Autodesk Inventor part; units mm, degrees
ref_plane "YZ Plane" through (0, 0, 0) normal (1, 0, 0) x (0, 1, 0)
ref_plane "XZ Plane" through (0, 0, 0) normal (0, 1, 0) x (-1, 0, 0)
ref_plane "XY Plane" through (0, 0, 0) normal (0, 0, 1) x (1, 0, 0)
sketch "Sketch1" plane through (0, 0, 0) normal (0, 0, 1) x (1, 0, 0)
  line L0 (0, 0) -> (0, 41.5)
  circle A0 centre (0, 41.5) radius 11
  line L1 (0, 41.5) -> (0, 52.5)
  line L2 (0, 52.5) -> (16, 52.5)
  line L3 (16, 52.5) -> (16, 0)
  line L4 (16, 0) -> (0, 0)
  line L5 (0, 0) -> (-16, 0)
  line L6 (-16, 0) -> (-16, 52.5)
  line L7 (-16, 52.5) -> (0, 52.5)
  dimension "d1" = 22
  dimension "d0" = 41.5
  dimension "d2" = 16
  dimension "d3" = 16
extrude "Extrusion1" add sketch "Sketch1" along normal mid plane 38
extrude "Extrusion2" add sketch "Sketch1" along normal mid plane 42 contours A0 L1 L0 | L0 L1 A0
fillet "Fillet1" radius 2 6 edges at (-16, 26.25, 19) (-16, 26.25, -19) (-16, 52.5, 0) (16, 52.5, 0) (16, 26.25, 19) (16, 26.25, -19)
sketch "Sketch2" plane through (-14, 0, 19) normal (0, -1, 0) x (1, 0, 0)
  circle A0 centre (14, -19) radius 11
  dimension "d9" = 22
extrude "Extrusion3" cut sketch "Sketch2" against normal blind 1
properties part number "Shoulder"
Verification items for the finished model (mm, model axes). A direction names the side the tool comes from. Coordinates: 2 decimals unless noted, no trailing zeros. Write each loop counter-clockwise with the first axis right and the second up, starting at its lowest first coordinate (ties: lowest second). Pieces come first, ordered by that corner, then holes. Notation, with made-up numbers: (24.25, 3) - (81.25, 3) arc R32 ccw to (81.25, 37) - close; hole circle Ø2 at (3, -27.75). An arc over 180 degrees is marked (long way). One line per question, with ' | ' between items. Start each with the question number.
1. Draft check along Z on faces 1 (the cylindrical face through (-15.43, 26.62, 18.4)), 2 (the flat face through (0, 1, 0)), 3 (the cylindrical face through (-15.4, 26.62, -18.43)), 4 (the flat face through (-7, 0, -9)). Enter one of: released by +Z, released by -Z, zero draft, split by the parting line, or undercut.
2. Section check C-C (y = 9.5). Enter the section's corners in (x, z), plus the area to 3 significant figures.
3. Section check A-A (y = 41.5). Enter the section's corners in (x, z).
4. Material ranges on line 1 along Z through (x, y) = (8, 24); line 2 along Y through (x, z) = (8.5, 3); line 3 along X through (y, z) = (41.5, -17.5), recorded low to high.
5. Gauge pin test, flat ends, axial feed: P1, Ø8.5, axis at x = 6.5, y = 21, coming from the -Z side; P2, Ø1, axis at x = 7, z = 1.5, coming from the -Y side; P3, Ø8, axis at x = 6.5, y = 9.5, coming from the +Z side. Record the tip position at first contact, or that the pin passes through.
6. Access from +Z, -Z, +X, -X, +Y, -Y to the whole of each face (thin tool, end or side, straight path). Record for faces 5 (the cylindrical face through (-2.38, 0.49, -10.74)), 6 (the cylindrical face through (-1.432, 52.406, 20.014)), 7 (the cylindrical face through (15.43, 25.88, 18.4)), 8 (the cylindrical face through (-1.432, 52.406, -19.986)), 9 (the cylindrical face through (15.4, 25.88, -18.43)).
7. Section check B-B (x = 4). Enter the section's corners in (y, z).
Computed values:
1) face 1: released by +Z | face 2: undercut | face 3: released by -Z | face 4: zero draft
2) outline: (-16, -17) arc R2 ccw to (-14, -19) - (14, -19) arc R2 ccw to (16, -17) - (16, 17) arc R2 ccw to (14, 19) - (-14, 19) arc R2 ccw to (-16, 17) - close | area: 1,210 mm²
3) outline: (-16, -17) arc R2 ccw to (-14, -19) - (-11, -19) - (-11, -21) - (11, -21) - (11, -19) - (14, -19) arc R2 ccw to (16, -17) - (16, 17) arc R2 ccw to (14, 19) - (11, 19) - (11, 21) - (-11, 21) - (-11, 19) - (-14, 19) arc R2 ccw to (-16, 17) - close
4) line 1: -19 to 19 | line 2: 1 to 52.5 | line 3: -15.94 to 15.94
5) P1: z = -19 | P2: y = 1 | P3: z = 19
6) face 5: -Y | face 6: +Z | face 7: +Z, +X, +Y, -Y | face 8: -Z | face 9: -Z, +X, +Y, -Y
7) outline: (0, -19) - (31.25, -19) - (31.25, -21) - (51.75, -21) - (51.75, -19) - (52.5, -19) - (52.5, 19) - (51.75, 19) - (51.75, 21) - (31.25, 21) - (31.25, 19) - (0, 19) - (0, 10.25) - (1, 10.25) - (1, -10.25) - (0, -10.25) - close
